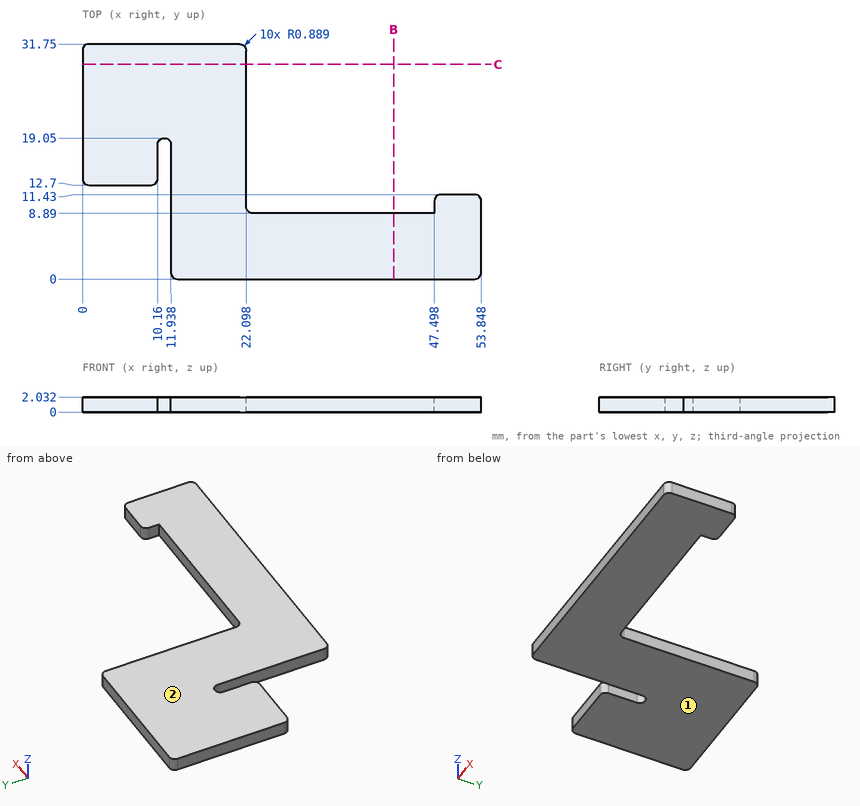
Drawing for the job (mm, zero at the part's lowest x, y, z). Coordinates: 2 decimals unless noted, no trailing zeros. Write each loop counter-clockwise with the first axis right and the second up, starting at its lowest first coordinate (ties: lowest second). Pieces come first, ordered by that corner, then holes. Notation, with made-up numbers: (-37.5, 34) - (11.5, 34) arc R30 ccw to (11.5, 64) - close; hole circle Ø6 at (48, 56). An arc over 180 degrees is marked (long way). Write each question's results on one line, items separated by ' | '. Start each with the question number.
1) Mould opens along Z. For the marked faces 1 and 2 say: pulls with the +Z half, pulls with the -Z half, needs draft (parallel to the pull), parting line crosses it, or undercut.
2) Cut at C-C (y = 29). Write the cut outline in (x, z), then the cut area to 3 significant figures.
3) Probe line 1 along X through (y, z) = (14.5, 0.1); line 2 along Y through (x, z) = (6, 0.6); line 3 along Y through (x, z) = (43.5, 0.4). List the from-to ranges inside material, lowest first. Write a range as from..to.
4) Cut at B-B (x = 42). Write the cut outline in (y, z), then the cut area to 3 significant figures.
5) Flat gauge pins, fed straight in: P1, Ø1, axis at y = 21, z = 1.5, coming from the +X side; P2, Ø1, axis at x = 5.5, z = 0.5, coming from the -Y side. Where does each tip first touch, or does it go through?
Returned:
1) face 1: pulls with the -Z half | face 2: pulls with the +Z half
2) outline: (0, 0) - (22.1, 0) - (22.1, 2.03) - (0, 2.03) - close | area: 44.9 mm^2
3) line 1: 0..10.16, 11.94..22.1 | line 2: 12.7..31.75 | line 3: 0..8.89
4) outline: (0, 0) - (8.89, 0) - (8.89, 2.03) - (0, 2.03) - close | area: 18.1 mm^2
5) P1: x = 22.1 | P2: y = 12.7
